from build123d import *

# Parameters (mm, degrees)
SKETCH_1_W          = 44.5
SKETCH_1_H          = 30
SKETCH_1_R          = 6.05
EXTRUDE_1_DEPTH     = 10
SKETCH_2_R          = 1.6
CUT_EXTRUDE_1_DEPTH = 10
SKETCH_3_R          = 2
CUT_EXTRUDE_2_DEPTH = 39.66603807


with BuildPart() as part:
    # ｽｹｯﾁ1 → ﾎﾞｽ - 押し出し1 (new body)
    with BuildSketch(Plane(origin=(0, 0, 0), x_dir=(0, 0, -1), z_dir=(1, 0, 0))):
        Rectangle(SKETCH_1_W, SKETCH_1_H)
        Circle(SKETCH_1_R, mode=Mode.SUBTRACT)
    extrude(amount=EXTRUDE_1_DEPTH)

    # ｽｹｯﾁ2 → ｶｯﾄ - 押し出し1 (cut)
    with BuildSketch(Plane.XY.offset(22.25)):
        with Locations((5, 10)):
            Circle(SKETCH_2_R)
        with Locations(Location((5, -10, 0), (0, 0, 180))):
            Circle(SKETCH_2_R)
    cut_extrude_1 = extrude(amount=-CUT_EXTRUDE_1_DEPTH, mode=Mode.SUBTRACT)

    # ｽｹｯﾁ3 → ｶｯﾄ - 押し出し2 (cut, through all)
    with BuildSketch(Plane(origin=(0, 15, 0), x_dir=(1, 0, 0), z_dir=(0, 1, 0))):
        with Locations(Location((5, 0, 0), (0, 0, 270))):
            Circle(SKETCH_3_R)
    extrude(amount=-CUT_EXTRUDE_2_DEPTH, mode=Mode.SUBTRACT)

    # ﾐﾗｰ1: ｶｯﾄ - 押し出し1 across plane
    add(cut_extrude_1.mirror(Plane.XY), mode=Mode.SUBTRACT)


solid = part.part
Input: part model. Units: mm. Frame: model coordinates. A direction names the side the tool comes from. Coordinates: 2 decimals unless noted, no trailing zeros. Loops run counter-clockwise (first coordinate to the right, second up) from the corner with the lowest first, then second, coordinate; pieces in that order, holes last. Notation, with made-up numbers: (-15, 0) -> (37, 0) arc R9 ccw to (37, 7) -> close; hole circle Ø6 at (24, -25.75). An arc over 180 degrees is marked (long way). Write each question's results on one line, items separated by ' | '. Start each with the question number.
Q1. Reachability of faces 1 (the cylindrical face through (4.65, 8.44, 17.32)), 2 (the flat face through (2.7, -15, 0.3)), 3 (the cylindrical face through (5.35, -8.44, -17.32)) from +Z, -Z, +X, -X, +Y, -Y: full face, straight path, thin tool, end or side. Return the list, or none.
Q2. Section C-C, the plane x = 8.75. Return the cut outline in (y, z).
Q3. Pin query (flat end, axial travel): pin 1 (14 mm diameter, centred on y = 0, z = 0, fed in from +X); pin 2 (2.5 mm diameter, centred on x = 5, y = 10, fed in from +Z); pin 3 (1.9 mm diameter, centred on x = 5, y = -10, fed in from -Z). Return the tip coordinate at first contact, or that it passes through.
Q4. Section D-D, the plane x = 4. Return the cut outline in (y, z), plus the area to 3 significant figures.
Q5. Section A-A, the plane y = 0. Return the cut outline in (x, z).
Q6. Ray query, line 1 (Y direction, x = 5, z = 15.75); line 2 (Y direction, x = 7.5, z = 2); line 3 (Y direction, x = 6.25, z = 14). Return the intervals inside material, ascending. Write a range as from..to.
Q7. Section B-B, the plane z = 0. Return the cut outline in (x, y), plus the area to 3 significant figures.
Q8. Pull-direction query (X, two-part tool) for faces 4 (the flat face through (5, 10, 12.25)), 5 (the flat face through (2.7, 15, 0.3)), 6 (the flat face through (10, 4, 5)), 7 (the flat face through (0, 4, 5)); classes: released by +X, released by -X, zero draft, split by the parting line, or undercut.
Found:
1) face 1: +Z | face 2: +Z, -Z, +X, -X, -Y | face 3: -Z
2) outline: (-15, -22.25) -> (15, -22.25) -> (15, 22.25) -> (-15, 22.25) -> close; hole circle Ø12.1 at (0, 0)
3) pin 1: x = 10 | pin 2: z = 12.25 | pin 3: z = -12.25
4) outline: (-15, -22.25) -> (-11.25, -22.25) -> (-11.25, -12.25) -> (-8.75, -12.25) -> (-8.75, -22.25) -> (8.75, -22.25) -> (8.75, -12.25) -> (11.25, -12.25) -> (11.25, -22.25) -> (15, -22.25) -> (15, -1.73) -> (5.8, -1.73) arc R6.05 cw to (-5.8, -1.73) -> (-15, -1.73) -> close; (-15, 1.73) -> (-5.8, 1.73) arc R6.05 cw to (5.8, 1.73) -> (15, 1.73) -> (15, 22.25) -> (11.25, 22.25) -> (11.25, 12.25) -> (8.75, 12.25) -> (8.75, 22.25) -> (-8.75, 22.25) -> (-8.75, 12.25) -> (-11.25, 12.25) -> (-11.25, 22.25) -> (-15, 22.25) -> close | area: 1,060 mm2
5) outline: (0, -22.25) -> (10, -22.25) -> (10, -6.05) -> (0, -6.05) -> close; (0, 6.05) -> (10, 6.05) -> (10, 22.25) -> (0, 22.25) -> close
6) line 1: -15..-11.6, -8.4..8.4, 11.6..15 | line 2: -15..-5.71, 5.71..15 | line 3: -15..-11, -9..9, 11..15
7) outline: (0, -15) -> (3, -15) -> (3, -6.05) -> (0, -6.05) -> close; (0, 6.05) -> (3, 6.05) -> (3, 15) -> (0, 15) -> close; (7, -15) -> (10, -15) -> (10, -6.05) -> (7, -6.05) -> close; (7, 6.05) -> (10, 6.05) -> (10, 15) -> (7, 15) -> close | area: 107 mm2
8) face 4: undercut | face 5: zero draft | face 6: released by +X | face 7: released by -X
